Geometry check sheet. Reference: the model listing, model coordinates, mm. Coordinates: 2 decimals unless noted, no trailing zeros. Write each loop counter-clockwise with the first axis right and the second up, starting at its lowest first coordinate (ties: lowest second). Pieces come first, ordered by that corner, then holes. Notation, with made-up numbers: M -23.75,-37 L -17.75,-37 A25 cw -17.75,-20 Z; hole C 67,85.5 d1. An arc over 180 degrees is marked long. Put each result on its own line as item: value. Start each with the question number.
1) Cross-section at A-A on z = 51. Record the cut outline in (x, y), plus the area to 3 significant figures.
2) Cross-section at B-B on y = -15. Record the cut outline in (x, z), plus the area to 4 significant figures.
3) Gauge pin test, flat ends, axial feed: pin 1 (1.5 mm diameter, centred on y = -33, z = 63, fed in from +X); pin 2 (5 mm diameter, centred on y = -43.5, z = 31.5, fed in from +X); pin 3 (3 mm diameter, centred on y = -35.5, z = 64.5, fed in from +X). Record the tip position at first contact, or that the pin passes through.
4) Scan lines: line 1 along X through (y, z) = (-22.5, 47); line 2 along X through (y, z) = (-8, 63); line 3 along Y through (x, z) = (1495, 30). Record each from-to range of solid material in increasing order.
from build123d import *

# Parameters (mm, degrees)
F0_W     = 1150
F0_H     = 50
F1_DEPTH = 50
F3_DEPTH = 25
F4_W     = 50
F4_H     = 50
F5_DEPTH = 25
F6_DEPTH = 25


with BuildPart() as f1:
    # F0 (on Front) → F1 (new body)
    with BuildSketch(Plane.XZ):
        with Locations((949.597177, 49.70942)):
            Rectangle(F0_W, F0_H)
        Polygon((1524.597177, 74.70942), (1524.597177, 24.70942), (1574.597177, 74.70942), align=None)
    extrude(amount=F1_DEPTH)

    # F2 (on face) → F3 (cut)
    with BuildSketch(Plane.XZ.offset(50)):
        Polygon((1524.597177, 24.70942), (1574.597177, 74.70942), (1503.886499, 74.70942), (1453.886499, 24.70942), align=None)
    extrude(amount=-F3_DEPTH, mode=Mode.SUBTRACT)

    # F4 (on face) → F5 (cut)
    with BuildSketch(Plane(origin=(0, 0, 0), x_dir=(-1, 0, 0), z_dir=(0, 1, 0))):
        with Locations((-399.597177, 49.70942)):
            Rectangle(F4_W, F4_H)
    extrude(amount=-F5_DEPTH, mode=Mode.SUBTRACT)

    # F2 (on face) → F6 (cut)
    with BuildSketch(Plane.XZ.offset(50)):
        Polygon((1524.597177, 24.70942), (1574.597177, 74.70942), (1503.886499, 74.70942), (1453.886499, 24.70942), align=None)
    extrude(amount=-F6_DEPTH, mode=Mode.SUBTRACT)


solid = f1.part
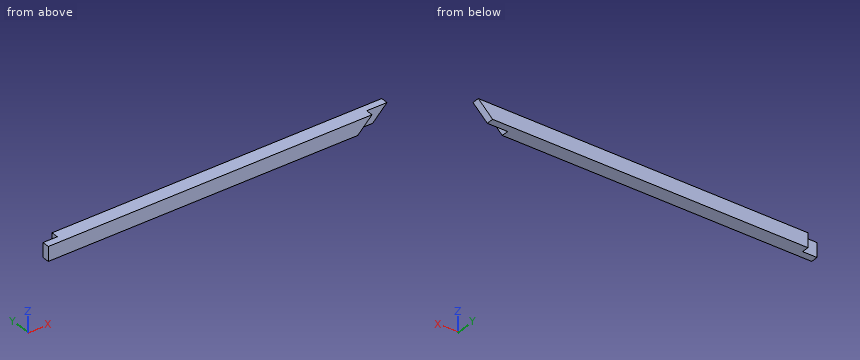
Answer key:
1. outline: M 374.6,-50 L 1480.18,-50 L 1480.18,-25 L 1550.89,-25 L 1550.89,0 L 424.6,0 L 424.6,-25 L 374.6,-25 Z
1. area: 55,800 mm²
2. outline: M 424.6,24.71 L 1524.6,24.71 L 1574.6,74.71 L 424.6,74.71 Z
2. area: 56,250 mm²
3. pin 1: stops at x = 1492.93
3. pin 2: stops at x = 1463.18
3. pin 3: stops at x = 1495.18
4. line 1: x = 424.6 to 1546.89
4. line 2: x = 424.6 to 1562.89
4. line 3: y = -25 to 0
